Geometry: final body of the model. Coordinates: model frame, mm. A direction names the side the tool comes from. Give positions to 0.01 mm unless a question says otherwise; leave off trailing zeros. Loops run counter-clockwise (first coordinate to the right, second up) from the corner with the lowest first, then second, coordinate; pieces in that order, holes last.
1. Material intervals for line 1 along Z through (x, y) = (23.5, 5); line 2 along X through (y, z) = (5.75, -8); line 3 along X through (y, z) = (2, -14), sorted ascending.
2. Section A-A, the plane y = 6.5. Output: boundary loops of the cut face in (x, z).
3. Section B-B, the plane z = -2. Output: boundary loops of the cut face in (x, y).
4. First-contact query: P1, Ø0.5, axis at y = 5.5, z = -6.5, coming from the -X side; P2, Ø15, axis at x = 19, z = -6.5, coming from the +Y side; P3, Ø2.5, axis at x = 2.5, y = 1.5, coming from the +Z side. Flat tips, straight axial feed; report the tip coordinate or a pass-through.
5. Draft query along Z for faces 1 (the face through (2, 2, -10)), 2 (the face through (39, 4, -5)), 3 (the face through (21.8, 5.5, -20.25)), 4 (the face through (37.74, 6.49, -4.77)). Return one class per face: +Z half, -Z half, draft (parallel to the pull), parting line (faces both ways), or undercut.
6. Section D-D, the plane y = 3.75. Output: boundary loops of the cut face in (x, z).
7. Access query for faces 5 (the face through (38.699, 3.958, -21.715)), 6 (the face through (6.75, 5.5, -4.8)), 7 (the face through (3, 5, -5)), 8 (the face through (3, 2, 0)). Directions: +Z, -Z, +X, -X, +Y, -Y. A direction counts if a zero-diameter tool reaches every point of the face in a straight line with its end or side. Return the directions, or none.
8. Section C-C, the plane x = 25.5. Output: boundary loops of the cut face in (y, z).
from build123d import *

# Parameters (mm, degrees)
EXTRUDE_1_DEPTH     = 5
SKETCH_2_W          = 34
SKETCH_2_H          = 34
EXTRUDE_2_DEPTH     = 2
SKETCH_3_W          = 30.5
SKETCH_3_H          = 30.5
CUT_EXTRUDE_2_DEPTH = 2.08
CHAMFER_1_SIZE      = 1
FILLET_2_R          = 1


with BuildPart() as part:
    # 草图1 → 凸台-拉伸1 (new body)
    with BuildSketch(Plane(origin=(0, 0, 0), x_dir=(1, 0, 0), z_dir=(0, 1, 0))):
        Polygon((0, 10), (5, 10), (5, 22), (39, 22), (39, -12), (5, -12), (5, 0), (0, 0), align=None)
    extrude(amount=EXTRUDE_1_DEPTH)

    # 草图2 → 凸台-拉伸2 (add)
    with BuildSketch(Plane(origin=(0, 5, 0), x_dir=(1, 0, 0), z_dir=(0, 1, 0))):
        with Locations((22, 5)):
            Rectangle(SKETCH_2_W, SKETCH_2_H)
    extrude(amount=EXTRUDE_2_DEPTH)

    # 草图3 → 切除-拉伸2 (cut)
    with BuildSketch(Plane(origin=(0, 7, 0), x_dir=(1, 0, 0), z_dir=(0, 1, 0))):
        with Locations((22, 5)):
            Rectangle(SKETCH_3_W, SKETCH_3_H)
    extrude(amount=-CUT_EXTRUDE_2_DEPTH, mode=Mode.SUBTRACT)

    # 倒角1
    chamfer_1_edges = [part.edges().sort_by_distance(p)[0] for p in [
        (22, 7, -20.25),
        (37.25, 7, -5),
        (22, 7, 10.25),
        (6.75, 7, -5),
    ]]
    chamfer(chamfer_1_edges, length=CHAMFER_1_SIZE)

    # 圆角2
    fillet_2_edges = [part.edges().sort_by_distance(p)[0] for p in [
        (5, 3.5, 12),
        (39, 3.5, 12),
        (39, 3.5, -22),
        (5, 3.5, -22),
        (22, 0, 12),
        (39, 0, -5),
        (22, 0, -22),
    ]]
    fillet(fillet_2_edges, radius=FILLET_2_R)


solid = part.part
Answers below:
1. line 1: z = -22 to -20.25, 10.25 to 12
1. line 2: x = 5 to 6.75, 37.25 to 39
1. line 3: x = 5 to 39
2. outline: (5, -21) arc R1 ccw to (6, -22) - (38, -22) arc R1 ccw to (39, -21) - (39, 11) arc R1 ccw to (38, 12) - (6, 12) arc R1 ccw to (5, 11) - close; hole (6.25, -20.75) - (37.75, -20.75) - (37.75, 10.75) - (6.25, 10.75) - close
3. outline: (0, 0) - (38, 0) arc R1 ccw to (39, 1) - (39, 7) - (38.25, 7) - (37.25, 6) - (37.25, 4.92) - (6.75, 4.92) - (6.75, 6) - (5.75, 7) - (5, 7) - (5, 5) - (0, 5) - close
4. P1: stops at x = 5
4. P2: stops at y = 4.92
4. P3: stops at z = 0
5. face 1: -Z half
5. face 2: draft
5. face 3: undercut
5. face 4: undercut
6. outline: (0, -10) - (5, -10) - (5, -21) arc R1 ccw to (6, -22) - (38, -22) arc R1 ccw to (39, -21) - (39, 11) arc R1 ccw to (38, 12) - (6, 12) arc R1 ccw to (5, 11) - (5, 0) - (0, 0) - close
7. face 5: -Z, +X, +Y, -Y
7. face 6: +Y
7. face 7: +Z, -Z, -X, +Y
7. face 8: +Z, -X, +Y, -Y
8. outline: (0, -21) arc R1 ccw to (1, -22) - (7, -22) - (7, -21.25) - (6, -20.25) - (4.92, -20.25) - (4.92, 10.25) - (6, 10.25) - (7, 11.25) - (7, 12) - (1, 12) arc R1 ccw to (0, 11) - close
